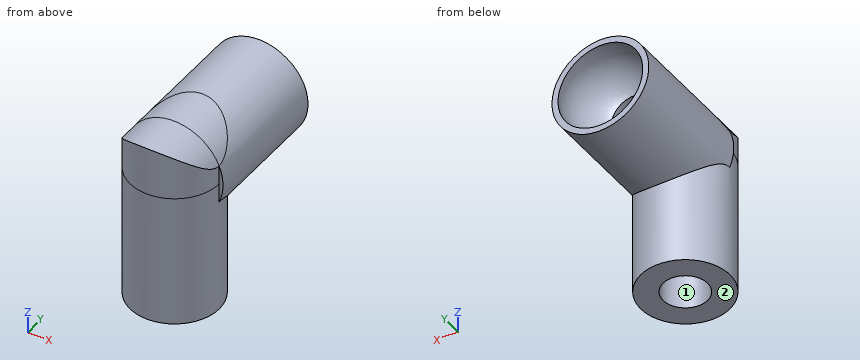
from build123d import *

# Parameters (mm, degrees)
SKETCH_5_R                       = 20
EXTRUDE_1_DEPTH                  = 60
EXTRUDE_1_DIRECTION_2_REACH      = 64.177
EXTRUDE_1_DIRECTION_2_END_RADIUS = 21.794494718
SKETCH_7_R                       = 10


with BuildPart() as part:
    # Sweep 1: sweep along a path in 草图2
    with BuildLine(Plane(origin=(0, 0, 0), x_dir=(1, 0, 0), z_dir=(0, 1, 0))) as sweep_1_path:
        CenterArc((0, 0), 11, 0, 360)
    # 草图1 → Sweep 1 (sweep)
    with BuildSketch(Plane.XY):
        with BuildLine():
            Line((21.794494718, 6), (21.794494718, -54))
            Line((21.794494718, -54), (0, -54))
            Line((0, -54), (0, -20))
            ThreePointArc((0, -20), (16.124515497, -11.832159566), (19.078784028, 6))
            Line((19.078784028, 6), (21.794494718, 6))
        make_face()
    sweep(path=sweep_1_path.line)

    # 草图5 → 凸台-拉伸1 (add)
    with BuildSketch(Plane.XY):
        with Locations((0, -54)):
            Circle(SKETCH_5_R)
    extrude(amount=-EXTRUDE_1_DEPTH)

    # 凸台-拉伸1 direction 2: up to this cylinder (the profile starts inside it)
    extrude_1_direction_2_end = Plane(origin=(0, -54, 0), z_dir=(0, 1, 0)) * Cylinder(EXTRUDE_1_DIRECTION_2_END_RADIUS, 172.942989435, mode=Mode.PRIVATE)
    # 草图5 → 凸台-拉伸1 direction 2 (add, up to the surface)
    with BuildSketch(Plane.XY, mode=Mode.PRIVATE) as extrude_1_direction_2_sk1:
        with Locations((0, -54)):
            Circle(SKETCH_5_R)
    extrude_1_direction_2_tool1 = extrude(extrude_1_direction_2_sk1.sketch, amount=EXTRUDE_1_DIRECTION_2_REACH, mode=Mode.PRIVATE) & extrude_1_direction_2_end
    add(extrude_1_direction_2_tool1.solids().sort_by_distance((0, -54, 0))[0])

    # Sweep 1 2: sweep along a path in 草图6
    with BuildLine(Plane(origin=(0, 0, 0), x_dir=(0, 0, -1), z_dir=(1, 0, 0))) as sweep_1_2_path:
        Line((60, -54), (0, -54))
        Line((0, -54), (0, 6))
    # 草图7 → Sweep 1 2 (sweep, cut)
    with BuildSketch(Plane(origin=(0, 0, -60), x_dir=(-1, 0, 0), z_dir=(0, 0, -1))):
        with Locations((0, -54)):
            Circle(SKETCH_7_R)
    sweep(path=sweep_1_2_path.line, transition=Transition.RIGHT, mode=Mode.SUBTRACT)


solid = part.part
Read the model definition and answer for the solid it produces. Units are mm, in the model's axes. Face numbers are marked on the shaded views. Round coordinates to 2 decimals unless told otherwise and drop trailing zeros. Loops run counter-clockwise (first coordinate to the right, second up) from the corner with the lowest first, then second, coordinate; pieces in that order, holes last.
Q1. Section A-A on z = -32.5 is taken. Write down the section's boundary in (x, y).
Q2. Consider probe 1 along Z at (x, y) = (0, -36); probe 2 along Y at (x, z) = (0, -46); probe 3 along X at (y, z) = (-54, -42.5). Determine where each line is inside the solid, lowest interval first.
Q3. Determine the mould class of the marked faces 1 and 2 for opening direction X: released by +X, released by -X, zero draft, split by the parting line, or undercut.
Q4. Each of these flat-tipped pins is pushed along its axis until it touches: pin 1 (8 mm diameter, centred on y = -48.5, z = 10, fed in from +X); pin 2 (12 mm diameter, centred on y = -38.5, z = 8.5, fed in from +X); pin 3 (16 mm diameter, centred on x = 0, z = 0, fed in from -Y); pin 4 (2 mm diameter, centred on x = 9.5, z = -31, fed in from -Y). Where does it stop, or does it pass through?
Q5. Section B-B on y = -40.5 is taken. Write down the section's boundary in (x, z).
Output:
1. outline: circle Ø40 at (0, -54); hole circle Ø20 at (0, -54)
2. probe 1: z = -60 to -10, 10 to 21.79
2. probe 2: y = -74 to -64, -44 to -34
2. probe 3: x = -20 to -10, 10 to 20
3. face 1: undercut
3. face 2: zero draft
4. pin 1: stops at x = 20.95
4. pin 2: stops at x = 21.65
4. pin 3: stops at y = -74
4. pin 4: stops at y = -72.1
5. outline: (-14.76, -60) - (14.76, -60) - (14.76, -16.04) arc R21.79 ccw (long way) to (-14.76, -16.04) - close; hole circle Ø20 at (0, 0)
